Verification items for the finished model (mm, model axes). A direction names the side the tool comes from. Round coordinates to 2 decimals unless told otherwise and drop trailing zeros. Loops run counter-clockwise (first coordinate to the right, second up) from the corner with the lowest first, then second, coordinate; pieces in that order, holes last. Notation, with made-up numbers: M -15.5,79 L 23.5,79 A33 ccw 23.5,110 Z; hole C -11.75,56.25 d7. An arc over 180 degrees is marked long. Answer as CSV lines item,"result".
```python
from build123d import *

# Parameters (mm, degrees)
SKETCH1_R           = 4.745
BASE_EXTRUDE_DEPTH  = 114.3
SKETCH2_R           = 3.175
BOSS_EXTRUDE1_DEPTH = 12.7
SKETCH3_R           = 4.745
SKETCH3_R_2         = 3.175
CUT_EXTRUDE1_DEPTH  = 15.875
CUT_EXTRUDE2_DEPTH  = 6.35


with BuildPart() as part:
    # Sketch1 → Base-Extrude (new body)
    with BuildSketch(Plane(origin=(0, 0, 0), x_dir=(0, 0, -1), z_dir=(1, 0, 0))):
        Circle(SKETCH1_R)
    extrude(amount=BASE_EXTRUDE_DEPTH)

    # Sketch2 → Boss-Extrude1 (add)
    with BuildSketch(Plane(origin=(114.3, 0, 0), x_dir=(0, 0, -1), z_dir=(1, 0, 0))):
        Circle(SKETCH2_R)
    extrude(amount=BOSS_EXTRUDE1_DEPTH)

    # Sketch3 → Cut-Extrude1 (cut)
    with BuildSketch(Plane.ZY):
        Circle(SKETCH3_R)
        with Locations(Location((0, 0, 0), (0, 0, 180))):
            Circle(SKETCH3_R_2, mode=Mode.SUBTRACT)
    extrude(amount=-CUT_EXTRUDE1_DEPTH, mode=Mode.SUBTRACT)

    # Sketch4 → Cut-Extrude2 (cut)
    with BuildSketch(Plane.ZY.offset(-15.875)):
        with BuildLine():
            Line((3.96875, 2.600778429), (3.96875, -2.600778429))
            ThreePointArc((3.96875, -2.600778429), (4.745, 0), (3.96875, 2.600778429))
        make_face()
        with BuildLine():
            Line((-3.96875, -2.600778429), (-3.96875, 2.600778429))
            ThreePointArc((-3.96875, 2.600778429), (-4.745, 0), (-3.96875, -2.600778429))
        make_face()
    extrude(amount=-CUT_EXTRUDE2_DEPTH, mode=Mode.SUBTRACT)


solid = part.part
```
1) Go/stop test with flat-tipped pins: pin 1 (2.5 mm diameter, centred on x = 19, y = -1, fed in from -Z); pin 2 (1.5 mm diameter, centred on x = 105, y = -3.5, fed in from -Z); pin 3 (4 mm diameter, centred on x = 20, y = 0, fed in from +Z). Record where each tip stops, or that it passes through.
Here are the results:
pin 1,"stops at z = -3.97"
pin 2,"stops at z = -3.87"
pin 3,"stops at z = 3.97"
2) Section check C-C (x = 37.5). Record the cut outline in (y, z) (3 decimals), plus the area to 3 significant figures.
Here are the results:
outline,"C 0,0 d9.49"
area,"70.7 mm^2"
3) Section check D-D (x = 17). Record the cut outline in (y, z) (3 decimals), plus the area to 3 significant figures.
Here are the results:
outline,"M -2.601,-3.969 L 2.601,-3.969 A4.745 ccw 2.601,3.969 L -2.601,3.969 A4.745 ccw Z"
area,"65.3 mm^2"
4) Material ranges on probe 1 along Y at (x, z) = (114.5, 0.25); probe 2 along X at (y, z) = (-1.25, 4.5) (3 decimals); probe 3 along X at (y, z) = (-3.25, -0.25) (3 decimals), recorded low to high.
Here are the results:
probe 1,"y = -3.17 to 3.17"
probe 2,"x = 22.225 to 114.3"
probe 3,"x = 15.875 to 114.3"
5) Set-up check for faces 4 (the flat face through (19, 0, -3.969)), 5 (the cylindrical face through (120.56, -3.1, 0.69)), 6 (the cylindrical face through (7.8, 2.8, -1.5)): record each of +Z, -Z, +X, -X, +Y, -Y from which the full face is reachable in a straight line by a thin tool's end or side.
Here are the results:
face 4,"-Z, -X, +Y, -Y"
face 5,"+X"
face 6,"-X"
6) Section check B-B (y = 0). Record the cut outline in (x, z) (3 decimals).
Here are the results:
outline,"M 0,-3.175 L 15.875,-3.175 L 15.875,-3.969 L 22.225,-3.969 L 22.225,-4.745 L 114.3,-4.745 L 114.3,-3.175 L 127,-3.175 L 127,3.175 L 114.3,3.175 L 114.3,4.745 L 22.225,4.745 L 22.225,3.969 L 15.875,3.969 L 15.875,3.175 L 0,3.175 Z"
7) Section check A-A (z = 0). Record the cut outline in (x, y) (3 decimals), plus the area to 3 significant figures.
Here are the results:
outline,"M 0,-3.175 L 15.875,-3.175 L 15.875,-4.745 L 114.3,-4.745 L 114.3,-3.175 L 127,-3.175 L 127,3.175 L 114.3,3.175 L 114.3,4.745 L 15.875,4.745 L 15.875,3.175 L 0,3.175 Z"
area,"1,120 mm^2"
8) Draft check along X on faces 1 (the flat face through (19, 0, 3.969)), 2 (the flat face through (127, 0, 0)), 3 (the flat face through (15.875, 3.23, 0.83)). Enter one of: +X half, -X half, draft (parallel to the pull), parting line (faces both ways), or undercut.
Here are the results:
face 1,"draft"
face 2,"+X half"
face 3,"-X half"
